from build123d import *

# Parameters (mm, degrees)
SKETCH1_W           = 95.25
SKETCH1_H           = 95.25
BOSS_EXTRUDE1_DEPTH = 152.4
SKETCH2_W           = 88.9
SKETCH2_H           = 44.45
CUT_EXTRUDE1_DEPTH  = 139.7
SKETCH2_3_W         = 88.9
SKETCH2_3_H         = 41.275
CUT_EXTRUDE2_DEPTH  = 111.76
SKETCH5_W           = 107.95
SKETCH5_H           = 107.95
SKETCH5_W_2         = 88.9
SKETCH5_H_2         = 88.9
BOSS_EXTRUDE2_DEPTH = 16.51
CUT_EXTRUDE5_DEPTH  = 16.51
SKETCH7_R           = 1.5
CUT_EXTRUDE6_DEPTH  = 7.874
SKETCH3_W           = 64.830855772
SKETCH3_H           = 22.015745463
SKETCH3_H_2         = 12.7
CUT_EXTRUDE7_DEPTH  = 30.48
SKETCH8_W           = 32.09515361
SKETCH8_H           = 4.475150354
CUT_EXTRUDE8_DEPTH  = 30.48


with BuildPart() as part:
    # Sketch1 → Boss-Extrude1 (new body)
    with BuildSketch(Plane.XY):
        Rectangle(SKETCH1_W, SKETCH1_H)
    extrude(amount=BOSS_EXTRUDE1_DEPTH)

    # Sketch2 → Cut-Extrude1 (cut)
    with BuildSketch(Plane.XY.offset(152.4)):
        with Locations((0, 22.225)):
            Rectangle(SKETCH2_W, SKETCH2_H)
    extrude(amount=-CUT_EXTRUDE1_DEPTH, mode=Mode.SUBTRACT)

    # Sketch2_3 → Cut-Extrude2 (cut)
    with BuildSketch(Plane.XY.offset(152.4)):
        with Locations((0, -23.8125)):
            Rectangle(SKETCH2_3_W, SKETCH2_3_H)
    extrude(amount=-CUT_EXTRUDE2_DEPTH, mode=Mode.SUBTRACT)

    # Sketch5 → Boss-Extrude2 (add)
    with BuildSketch(Plane.XY.offset(152.4)):
        Rectangle(SKETCH5_W, SKETCH5_H)
        Rectangle(SKETCH5_W_2, SKETCH5_H_2, mode=Mode.SUBTRACT)
    extrude(amount=-BOSS_EXTRUDE2_DEPTH)

    # Sketch6 → Cut-Extrude5 (cut)
    with BuildSketch(Plane.XY.offset(152.4)):
        with BuildLine():
            Line((-50.8, 49.3), (-50.8, 50.8))
            Line((-50.8, 50.8), (-49.3, 50.8))
            ThreePointArc((-49.3, 50.8), (-51.860660172, 51.860660172), (-50.8, 49.3))
        make_face()
        with BuildLine():
            Line((-49.3, 50.8), (-50.8, 50.8))
            Line((-50.8, 50.8), (-50.8, 49.3))
            ThreePointArc((-50.8, 49.3), (-49.739339828, 49.739339828), (-49.3, 50.8))
        make_face()
        with BuildLine():
            ThreePointArc((52.3, 50.8), (50.8, 52.3), (49.3, 50.8))
            Line((49.3, 50.8), (50.8, 50.8))
            Line((50.8, 50.8), (50.8, 49.3))
            ThreePointArc((50.8, 49.3), (51.860660172, 49.739339828), (52.3, 50.8))
        make_face()
        with BuildLine():
            Line((50.8, 50.8), (49.3, 50.8))
            ThreePointArc((49.3, 50.8), (49.739339828, 49.739339828), (50.8, 49.3))
            Line((50.8, 49.3), (50.8, 50.8))
        make_face()
        with BuildLine():
            ThreePointArc((-49.3, -50.8), (-49.739339828, -49.739339828), (-50.8, -49.3))
            Line((-50.8, -49.3), (-50.8, -50.8))
            Line((-50.8, -50.8), (-49.3, -50.8))
        make_face()
        with BuildLine():
            Line((-50.8, -50.8), (-50.8, -49.3))
            ThreePointArc((-50.8, -49.3), (-51.860660172, -51.860660172), (-49.3, -50.8))
            Line((-49.3, -50.8), (-50.8, -50.8))
        make_face()
        with BuildLine():
            ThreePointArc((52.3, -50.8), (51.860660172, -49.739339828), (50.8, -49.3))
            Line((50.8, -49.3), (50.8, -50.8))
            Line((50.8, -50.8), (49.3, -50.8))
            ThreePointArc((49.3, -50.8), (50.8, -52.3), (52.3, -50.8))
        make_face()
        with BuildLine():
            Line((50.8, -50.8), (50.8, -49.3))
            ThreePointArc((50.8, -49.3), (49.739339828, -49.739339828), (49.3, -50.8))
            Line((49.3, -50.8), (50.8, -50.8))
        make_face()
    extrude(amount=-CUT_EXTRUDE5_DEPTH, mode=Mode.SUBTRACT)

    # Sketch7 → Cut-Extrude6 (cut)
    with BuildSketch(Plane(origin=(0, 0, 0), x_dir=(-1, 0, 0), z_dir=(0, 0, -1))):
        with Locations((-44.45, 0.987495031)):
            Circle(SKETCH7_R)
        with Locations((44.45, 0.987495031)):
            Circle(SKETCH7_R)
        with Locations((44.45, -42.992427459)):
            Circle(SKETCH7_R)
        with Locations((-44.45, -42.992427459)):
            Circle(SKETCH7_R)
    extrude(amount=-CUT_EXTRUDE6_DEPTH, mode=Mode.SUBTRACT)

    # Sketch3 → Cut-Extrude7 (cut)
    with BuildSketch(Plane(origin=(0, 0, 0), x_dir=(-1, 0, 0), z_dir=(0, 0, -1))):
        Polygon((41.787446397, -3.204523257), (-42.032553603, -3.204523257), (-42.032553603, -31.144523257), (-32.415427886, -31.144523257), (-32.415427886, -9.128777794), (32.415427886, -9.128777794), (32.415427886, -31.144523257), (41.787446397, -31.144523257), align=None)
        with Locations((0, -20.136650526)):
            Rectangle(SKETCH3_W, SKETCH3_H)
        with Locations((0, -37.494523257)):
            Rectangle(SKETCH3_W, SKETCH3_H_2)
    extrude(amount=-CUT_EXTRUDE7_DEPTH, mode=Mode.SUBTRACT)

    # Sketch8 → Cut-Extrude8 (cut)
    with BuildSketch(Plane(origin=(0, 0, 30.48), x_dir=(-1, 0, 0), z_dir=(0, 0, -1))):
        with Locations((0, -41.60694808)):
            Rectangle(SKETCH8_W, SKETCH8_H)
    extrude(amount=-CUT_EXTRUDE8_DEPTH, mode=Mode.SUBTRACT)


solid = part.part
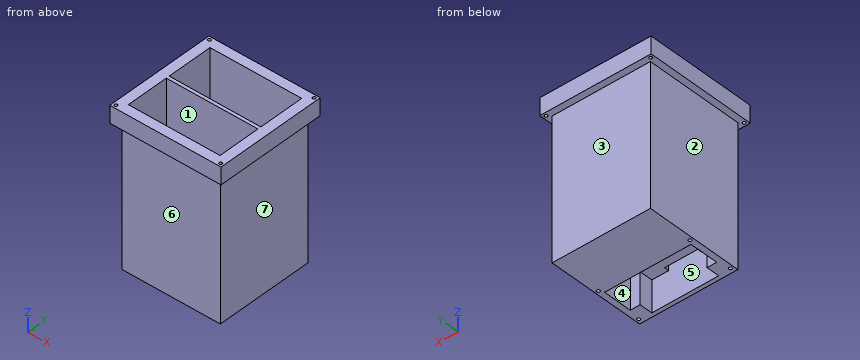
For this review, take the finished solid that the model builds, in its own axes (mm). Face numbers are marked on the shaded views. A direction names the side the tool comes from. Give positions to 0.01 mm unless a question says otherwise; leave off trailing zeros. Loops run counter-clockwise (first coordinate to the right, second up) from the corner with the lowest first, then second, coordinate; pieces in that order, holes last. Notation, with made-up numbers: M 33,65 L 69,65 A24 ccw 69,102 Z; hole C 57,17 d10. An arc over 180 degrees is marked long. Answer as a JSON object with one key per item and string values. Group by question number.
Q1. Mouldability with a two-part tool opening along X and no side actions: class the marked faces 5, 6 and 7 as +X half, -X half, draft (parallel to the pull), parting line (faces both ways), or undercut.
Q2. For probe 1 along X at (y, z) = (-50.8, 148) (3 decimals); probe 2 along Y at (x, z) = (-12.5, 132) (3 decimals); probe 3 along Y at (x, z) = (-44.45, 2.75) (1 decimal), list the stretches that pass through material, from the lowest coordinate up. Write a range as [from, to].
Q3. Add section B-B on y = 41.5. Give the boundary of the cut face in (x, z) (3 decimals).
Q4. Add section A-A on x = 2.5. Give the boundary of the cut face in (y, z) (3 decimals), and give its area (3 significant figures).
Q5. Insertion check: P1, Ø6, axis at x = 16.5, y = -22, coming from the -Z side; P2, Ø6, axis at y = -14, z = 86, coming from the -X side (3 decimals); P3, Ø2, axis at x = 10.5, z = 36.5, coming from the -Y side (3 decimals). Each pin has a flat end and moves straight along its axis. Give the tip position at first contact, or say it passes through.
Q6. Add section C-C on z = 122.5. Give the boundary of the cut face in (x, y) (3 decimals).
Q7. Add section D-D on x = -26.5. Give the boundary of the cut face in (y, z) (3 decimals).
Q8. Tool access review of the marked faces 1, 2, 3 and 4: name each direction out of +Z, -Z, +X, -X, +Y, -Y from which nothing blocks a thin tool from reaching the whole face with its end or side.
Checked values:
{
 "1": {"face 5": "undercut", "face 6": "draft", "face 7": "+X half"},
 "2": {"probe 1": "[-53.975, -52.3], [-49.3, 49.3], [52.3, 53.975]", "probe 2": "[-47.625, -44.45], [-3.175, 0], [44.45, 47.625]", "probe 3": "[-47.6, -44.5], [-41.5, -0.5], [2.5, 47.6]"},
 "3": {"outline": "M -53.975,135.89 L -47.625,135.89 L -47.625,0 L 47.625,0 L 47.625,135.89 L 53.975,135.89 L 53.975,152.4 L 44.45,152.4 L 44.45,12.7 L -44.45,12.7 L -44.45,152.4 L -53.975,152.4 Z"},
 "4": {"outline": "M -53.975,135.89 L -47.625,135.89 L -47.625,0 L -43.845,0 L -43.845,40.64 L -44.45,40.64 L -44.45,152.4 L -53.975,152.4 Z; M -39.369,30.48 L -3.205,30.48 L -3.205,0 L 47.625,0 L 47.625,135.89 L 53.975,135.89 L 53.975,152.4 L 44.45,152.4 L 44.45,12.7 L 0,12.7 L 0,152.4 L -3.175,152.4 L -3.175,40.64 L -39.369,40.64 Z", "area": "2,620 mm²"},
 "5": {"P1": "z = 30.48", "P2": "x = -47.625", "P3": "y = -47.625"},
 "6": {"outline": "M -47.625,-47.625 L 47.625,-47.625 L 47.625,47.625 L -47.625,47.625 Z; hole M -44.45,-44.45 L 44.45,-44.45 L 44.45,-3.175 L -44.45,-3.175 Z; hole M -44.45,0 L 44.45,0 L 44.45,44.45 L -44.45,44.45 Z"},
 "7": {"outline": "M -53.975,135.89 L -47.625,135.89 L -47.625,0 L -43.845,0 L -43.845,30.48 L -3.205,30.48 L -3.205,0 L 47.625,0 L 47.625,135.89 L 53.975,135.89 L 53.975,152.4 L 44.45,152.4 L 44.45,12.7 L 0,12.7 L 0,152.4 L -3.175,152.4 L -3.175,40.64 L -44.45,40.64 L -44.45,152.4 L -53.975,152.4 Z"},
 "8": {"face 1": "+Z", "face 2": "-Z, -X, +Y, -Y", "face 3": "-Z, +X, -X, +Y", "face 4": "-Z"}
}
